from build123d import *

# Parameters (mm, degrees)
F1_DEPTH = 508


with BuildPart() as f1:
    # F0 (on Front) → F1 (new body)
    with BuildSketch(Plane.XZ):
        with BuildLine():
            ThreePointArc((-21.52567, 4.242823), (-18.903543, 6.585581), (-17.929995, 9.964378))
            ThreePointArc((-17.929995, 9.964378), (-27.658792, 15.34083), (-27.034319, 4.242823))
            ThreePointArc((-27.034319, 4.242823), (-24.279995, 3.614378), (-21.52567, 4.242823))
        make_face()
        with BuildLine():
            ThreePointArc((-21.52567, 4.242823), (-24.279995, 3.614378), (-27.034319, 4.242823))
            Line((-27.034319, 4.242823), (-33.804995, -6.501848))
            Line((-33.804995, -6.501848), (-24.279995, -6.501848))
            Line((-24.279995, -6.501848), (-14.754995, -6.501848))
            Line((-14.754995, -6.501848), (-21.52567, 4.242823))
        make_face()
        Polygon((-24.279995, -6.501848), (-33.804995, -6.501848), (-43.329995, -6.501848), (-43.329995, -12.851848), (-5.229995, -12.851848), (-5.229995, -6.501848), (-14.754995, -6.501848), align=None)
    extrude(amount=F1_DEPTH)


solid = f1.part
Design review of the part built by this model. Coordinates are the model's own, in mm. A direction names the side the tool comes from. Round coordinates to 2 decimals unless told otherwise and drop trailing zeros. Order: outer loops, then holes, each group sorted by start corner. A loop starts at its lowest first (then second) coordinate and runs counter-clockwise, first axis right, second up. Notation, with made-up numbers: M -13.75,7.25 L 5.25,7.25 A28 ccw 5.25,40.25 Z; hole C -29,37.5 d4. An arc over 180 degrees is marked long. Answer as CSV lines item,"result". Start each with the question number.
1) Add section A-A (y = -402). Give the boundary of the cut face in (x, z) (3 decimals).
2) Wall thickness on line 1 along Z through (x, y) = (-33, -348); line 2 along Z through (x, y) = (-10, -173); line 3 along Z through (x, y) = (-18.5, -306): over which ranges is each line inside the solid? List them lowest first. Write a range as [from, to].
3) For pin 1 Ø1 at (y, z) = (-173.5, -3.5) entering from +X; pin 2 Ø7.5 at (x, y) = (-12, -188) entering from +Z; pin 3 Ø3 at (y, z) = (-143.5, 1.5) entering from -X, all flat-tipped, find the tip position at first contact; note any pin that passes through.
4) The part is to be moulded in two halves that separate along Z. For faces 1 (the face through (-25, -250, -12.852)), 2 (the face through (-39, -250, -6.502)), 3 (the face through (-25, 0, -1)), 4 (the face through (-18.093, -250.444, -1.205)), say which applies: +Z half, -Z half, draft (parallel to the pull), parting line (faces both ways), or undercut.
5) Tool access review of faces 5 (the face through (-25, -508, -1)), 6 (the face through (-30.4, -250.4, -1.1)), 7 (the face through (-10, -250, -6.502)): name each direction out of +Z, -Z, +X, -X, +Y, -Y from which nothing blocks a thin tool from reaching the whole face with its end or side.
Resolved:
1,outline,"M -43.33,-12.852 L -5.23,-12.852 L -5.23,-6.502 L -14.755,-6.502 L -21.526,4.243 A6.35 ccw -17.93,9.964 A6.35 ccw long -27.034,4.243 L -33.805,-6.502 L -43.33,-6.502 Z"
2,line 1,"[-12.85, -5.22]"
2,line 2,"[-12.85, -6.5]"
2,line 3,"[-12.85, -0.56], [7.33, 12.59]"
3,pin 1,"x = -16.33"
3,pin 2,"z = -4.92"
3,pin 3,"x = -29.71"
4,face 1,"-Z half"
4,face 2,"+Z half"
4,face 3,"draft"
4,face 4,"undercut"
5,face 5,"+Z, -Z, +X, -X, -Y"
5,face 6,"-X, +Y, -Y"
5,face 7,"+Z, +X, +Y, -Y"
